```python
from build123d import *

# Parameters (mm, degrees)
F2_T = -2.54


with BuildPart() as f1:
    # F0 (on Front) → F1 (revolve)
    with BuildSketch(Plane.XZ):
        with BuildLine():
            Line((31.75, 0), (0, 0))
            Line((0, 0), (0, -38.1))
            Line((0, -38.1), (25.4, -38.1))
            ThreePointArc((25.4, -38.1), (29.890128, -36.240128), (31.75, -31.75))
            Line((31.75, -31.75), (31.75, 0))
        make_face()
    revolve(axis=Axis((0, 0, -6.767765), (0, 0, -1)))

    # F2
    f2_openings = [f1.faces().sort_by_distance(p)[0] for p in [
        (0, 0, 0),
    ]]
    offset(amount=F2_T, openings=f2_openings)


solid = f1.part
```
For this review, take the finished solid that the model builds, in its own axes (mm). A direction names the side the tool comes from. Round coordinates to 2 decimals unless told otherwise and drop trailing zeros. Write each loop counter-clockwise with the first axis right and the second up, starting at its lowest first coordinate (ties: lowest second). Pieces come first, ordered by that corner, then holes. Notation, with made-up numbers: (-1, 72) - (3, 72) arc R21 ccw to (3, 106) - close; hole circle Ø11 at (-31, 56). An arc over 180 degrees is marked (long way). Answer as CSV lines item,"result". Start each with the question number.
(1) For line 1 (X direction, y = -1, z = -29); line 2 (Y direction, x = 0, z = -18); line 3 (Z direction, x = -7.5, y = -18.5), list the stretches that pass through material, from the lowest coordinate up.
(2) Add section A-A, the plane z = -7. State the section outline as (x, y) points.
(3) Machinability: for faces 1 (the flat face through (0, 0, -38.1)), 2 (the cylindrical face through (-21.53, -19.74, -15.65)), which of the approach directions +Z, -Z, +X, -X, +Y, -Y give a long, thin tool a straight path to every point of the face, cutting with its end or side? Answer none if there is none.
(4) For pin 1 (5 mm diameter, centred on y = -18, z = -20, fed in from +X); pin 2 (5 mm diameter, centred on y = -11.5, z = -13, fed in from +X); pin 3 (10 mm diameter, centred on y = 21, z = -20.5, fed in from +X), all flat-tipped, find the tip position at first contact; note any pin that passes through.
(5) Mouldability with a two-part tool opening along Y and no side actions: class faces 3 (the cylindrical face through (-6.883, 30.995, -15.653)), 4 (the flat face through (0, 0, -35.56)), 5 (the flat face through (14, 26, 0)) as +Y half, -Y half, draft (parallel to the pull), parting line (faces both ways), or undercut.
(6) Add section B-B, the plane x = 0. State the section outline as (y, z) points.
From the geometry:
1,line 1,"x = -31.73 to -29.19, 29.19 to 31.73"
1,line 2,"y = -31.75 to -29.21, 29.21 to 31.75"
1,line 3,"z = -38.1 to -35.56"
2,outline,"circle Ø63.5 at (0, 0); hole circle Ø58.42 at (0, 0)"
3,face 1,"-Z, +X, -X, +Y, -Y"
3,face 2,"+Z"
4,pin 1,"stops at x = 27.71"
4,pin 2,"stops at x = 30.45"
4,pin 3,"stops at x = 27.42"
5,face 3,"parting line"
5,face 4,"undercut"
5,face 5,"draft"
6,outline,"(-31.75, -31.75) arc R6.35 ccw to (-25.4, -38.1) - (25.4, -38.1) arc R6.35 ccw to (31.75, -31.75) - (31.75, 0) - (29.21, 0) - (29.21, -31.75) arc R3.81 cw to (25.4, -35.56) - (-25.4, -35.56) arc R3.81 cw to (-29.21, -31.75) - (-29.21, 0) - (-31.75, 0) - close"
